Read the model definition and answer for the solid it produces. Units are mm, in the model's axes. Coordinates: 2 decimals unless noted, no trailing zeros. Write each loop counter-clockwise with the first axis right and the second up, starting at its lowest first coordinate (ties: lowest second). Pieces come first, ordered by that corner, then holes. Notation, with made-up numbers: (-17, -38) - (30, -38) arc R21 cw to (30, -19) - close; hole circle Ø5 at (55.5, 58.25). An arc over 180 degrees is marked (long way). Return JSON: item names as keys, results as strings.
```python
from build123d import *

# Parameters (mm, degrees)
BOSS_EXTRUDE1_DEPTH     = 6.35
F_1_2_CLEARANCE_HOLE1_D = 13.49248


with BuildPart() as part:
    # Sketch1 → Boss-Extrude1 (new, symmetric)
    with BuildSketch(Plane.XY):
        Polygon((0, 0), (0, 203.2), (50.957425301, 203.2), (168.275, 0), align=None)
    extrude(amount=BOSS_EXTRUDE1_DEPTH, both=True)

    # 1/2 Clearance Hole1 (through all)
    with Locations(Plane.XY.offset(6.35)):
        with Locations((44.45, 101.6)):
            Hole(F_1_2_CLEARANCE_HOLE1_D / 2)


solid = part.part
```
(1) Straight lines are drawn through the part: line 1 (Y direction, x = 44.45, z = 2.75); line 2 (Y direction, x = 49.5, z = 4.25); line 3 (X direction, y = 98.5, z = 0.75). For each, find the intervals that lie inside material, in ascending order. Write a range as from..to.
Answer:
{"line 1": "0..94.85, 108.35..203.2", "line 2": "0..97.13, 106.07..203.2", "line 3": "0..38.46, 50.44..111.41"}
(2) A cutting plane is placed at A-A (x = 44.45). Determine the outline of the cut face in (y, z), and give its area (3 significant figures).
Answer:
{"outline": "(0, -6.35) - (94.85, -6.35) - (94.85, 6.35) - (0, 6.35) - close; (108.35, -6.35) - (203.2, -6.35) - (203.2, 6.35) - (108.35, 6.35) - close", "area": "2,410 mm²"}
(3) Flat-ended cylindrical pins translate along their axes: P1, Ø3, axis at y = 105, z = -4, coming from the +X side; P2, Ø2, axis at y = 177.5, z = -3, coming from the +X side; P3, Ø3, axis at x = 104, z = -2.5, coming from the +Y side. Find the tip coordinate at first contact, or state that the pin passes through.
Answer:
{"P1": "x = 108.52", "P2": "x = 66.37", "P3": "y = 113.93"}
(4) A cutting plane is placed at C-C (y = 101.6). Determine the outline of the cut face in (x, z), and give its area (3 significant figures).
Answer:
{"outline": "(0, -6.35) - (37.7, -6.35) - (37.7, 6.35) - (0, 6.35) - close; (51.2, -6.35) - (109.62, -6.35) - (109.62, 6.35) - (51.2, 6.35) - close", "area": "1,220 mm²"}
(5) Determine the mould class of faces 1 (the face through (108.795, 103.022, 0.089)), 2 (the face through (25, 203.2, 0)), 3 (the face through (49.42, 106.16, -0.09)), 4 (the face through (0, 100, 0)) for opening direction X: +X half, -X half, draft (parallel to the pull), parting line (faces both ways), or undercut.
Answer:
{"face 1": "+X half", "face 2": "draft", "face 3": "undercut", "face 4": "-X half"}
(6) A cutting plane is placed at D-D (x = 91). Determine the outline of the cut face in (y, z).
Answer:
{"outline": "(0, -6.35) - (133.84, -6.35) - (133.84, 6.35) - (0, 6.35) - close"}
(7) A cutting plane is placed at B-B (z = 0.25). Determine the outline of the cut face in (x, y) (3 decimals).
Answer:
{"outline": "(0, 0) - (168.275, 0) - (50.957, 203.2) - (0, 203.2) - close; hole circle Ø13.492 at (44.45, 101.6)"}
